Geometry check sheet. Reference: the model listing, model coordinates, mm. Face numbers are marked on the shaded views. Round coordinates to 2 decimals unless told otherwise and drop trailing zeros. Write each loop counter-clockwise with the first axis right and the second up, starting at its lowest first coordinate (ties: lowest second). Pieces come first, ordered by that corner, then holes. Notation, with made-up numbers: M 47.25,76.25 L 87.25,76.25 A18 ccw 87.25,89.25 Z; hole C -37,88 d2. An arc over 180 degrees is marked long. Use a Markdown table: item, result.
```python
from build123d import *

# Parameters (mm, degrees)
SKETCH1_W           = 58
SKETCH1_H           = 30.5
BOSS_EXTRUDE1_DEPTH = 3.5
SKETCH2_R           = 5.077771543
BOSS_EXTRUDE2_DEPTH = 5.9
SKETCH3_W           = 79
SKETCH3_H           = 30
BOSS_EXTRUDE3_DEPTH = 1.8
SKETCH4_R           = 7.569009477
BOSS_EXTRUDE4_DEPTH = 2.5
SKETCH5_W           = 65
SKETCH5_H           = 30
BOSS_EXTRUDE5_DEPTH = 1.5
SKETCH6_W           = 11.5
SKETCH6_H           = 7.5
SKETCH6_W_2         = 7.5
SKETCH6_H_2         = 5.5
BOSS_EXTRUDE6_DEPTH = 3.5


with BuildPart() as part:
    # Sketch1 → Boss-Extrude1 (new body)
    with BuildSketch(Plane.XY):
        Rectangle(SKETCH1_W, SKETCH1_H)
    extrude(amount=BOSS_EXTRUDE1_DEPTH)

    # Sketch2 → Boss-Extrude2 (add)
    with BuildSketch(Plane.XY.offset(3.5)):
        Circle(SKETCH2_R)
    extrude(amount=BOSS_EXTRUDE2_DEPTH)

    # Sketch3 → Boss-Extrude3 (add)
    with BuildSketch(Plane.XY.offset(9.4)):
        with Locations((0.5, 0.5)):
            Rectangle(SKETCH3_W, SKETCH3_H)
    extrude(amount=BOSS_EXTRUDE3_DEPTH)

    # Sketch4 → Boss-Extrude4 (add)
    with BuildSketch(Plane(origin=(0, 0, 11.2), x_dir=(-1, 0, 0), z_dir=(0, 0, -1))):
        Circle(SKETCH4_R)
    extrude(amount=-BOSS_EXTRUDE4_DEPTH)

    # Sketch5 → Boss-Extrude5 (add)
    with BuildSketch(Plane(origin=(0, 0, 13.7), x_dir=(-1, 0, 0), z_dir=(0, 0, -1))):
        Rectangle(SKETCH5_W, SKETCH5_H)
    extrude(amount=-BOSS_EXTRUDE5_DEPTH)

    # Sketch6 → Boss-Extrude6 (add)
    with BuildSketch(Plane.XY.offset(15.2)):
        with Locations((-20.25, -12.25)):
            Rectangle(SKETCH6_W, SKETCH6_H)
        with Locations((21.25, -13.25)):
            Rectangle(SKETCH6_W_2, SKETCH6_H_2)
        with Locations((8.75, -13.25)):
            Rectangle(SKETCH6_W_2, SKETCH6_H_2)
    extrude(amount=BOSS_EXTRUDE6_DEPTH)


solid = part.part
```
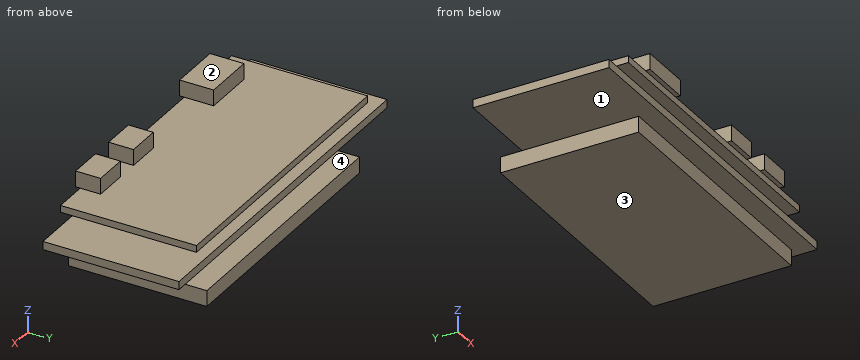
Item 1: Cross-section at A-A, the plane y = 9.5. Record the cut outline in (x, z), and give its area (3 significant figures).
Outcome:
| item | result |
|---|---|
| outline | M -39,9.4 L 40,9.4 L 40,11.2 L -39,11.2 Z; M -32.5,13.7 L 32.5,13.7 L 32.5,15.2 L -32.5,15.2 Z; M -29,0 L 29,0 L 29,3.5 L -29,3.5 Z |
| area | 443 mm2 |
Item 2: Cross-section at C-C, the plane x = 21. Record the cut outline in (y, z), and give its area (3 significant figures).
Outcome:
| item | result |
|---|---|
| outline | M -16,15.2 L -15,15.2 L -15,13.7 L 15,13.7 L 15,15.2 L -10.5,15.2 L -10.5,18.7 L -16,18.7 Z; M -15.25,0 L 15.25,0 L 15.25,3.5 L -15.25,3.5 Z; M -14.5,9.4 L 15.5,9.4 L 15.5,11.2 L -14.5,11.2 Z |
| area | 225 mm2 |
Item 3: Cross-section at B-B, the plane z = 16.5. Record the cut outline in (x, y), and give its area (3 significant figures).
Outcome:
| item | result |
|---|---|
| outline | M -26,-16 L -14.5,-16 L -14.5,-8.5 L -26,-8.5 Z; M 5,-16 L 12.5,-16 L 12.5,-10.5 L 5,-10.5 Z; M 17.5,-16 L 25,-16 L 25,-10.5 L 17.5,-10.5 Z |
| area | 169 mm2 |
Item 4: Material ranges on line 1 along X through (y, z) = (-12, 16.25); line 2 along Z through (x, y) = (15.5, 5.5); line 3 along Z through (x, y) = (11, -14), recorded low to high. Write a range as from..to.
Outcome:
| item | result |
|---|---|
| line 1 | x = -26..-14.5, 5..12.5, 17.5..25 |
| line 2 | z = 0..3.5, 9.4..11.2, 13.7..15.2 |
| line 3 | z = 0..3.5, 9.4..11.2, 13.7..18.7 |
Item 5: Go/stop test with flat-tipped pins: pin 1 (2 mm diameter, centred on x = 29.5, z = 3, fed in from +Y); pin 2 (1 mm diameter, centred on x = -12, z = 16, fed in from +Y); pin 3 (4 mm diameter, centred on x = 21.5, z = 16.5, fed in from +Y); pin 4 (0.5 mm diameter, centred on x = 3, z = 10.5, fed in from -Y). Record where each tip stops, or that it passes through.
Outcome:
| item | result |
|---|---|
| pin 1 | stops at y = 15.25 |
| pin 2 | passes through |
| pin 3 | stops at y = 15 |
| pin 4 | stops at y = -14.5 |
Item 6: Cross-section at D-D, the plane x = 31. Record the cut outline in (y, z).
Outcome:
| item | result |
|---|---|
| outline | M -15,13.7 L 15,13.7 L 15,15.2 L -15,15.2 Z; M -14.5,9.4 L 15.5,9.4 L 15.5,11.2 L -14.5,11.2 Z |
Item 7: Mould release check, pull along Z, two halves, no side actions. Record for the marked faces 1, 2, 3 and 4: +Z half, -Z half, draft (parallel to the pull), parting line (faces both ways), or undercut.
Outcome:
| item | result |
|---|---|
| face 1 | undercut |
| face 2 | +Z half |
| face 3 | -Z half |
| face 4 | undercut |
